from build123d import *

# Parameters (mm, degrees)
BOSS_EXTRUDE3_DEPTH = 4
SKETCH2_W           = 40
SKETCH2_H           = 36.696145016
SKETCH2_W_2         = 20
SKETCH2_H_2         = 40
BOSS_EXTRUDE4_DEPTH = 2
LOFT8_START         = -60
LOFT8_DEPTH         = 40
SKETCH10_W          = 24
SKETCH10_H          = 13
CUT_EXTRUDE1_DEPTH  = 6
SKETCH11_W          = 20
SKETCH11_H          = 40
BOSS_EXTRUDE5_DEPTH = 4


# Read off the part's stored shape, not the designer's step: Loft8
with BuildPart() as part:
    # Sketch1 → Boss-Extrude3 (new body)
    with BuildSketch(Plane(origin=(0, 0, 0), x_dir=(1, 0, 0), z_dir=(0, 1, 0))):
        with BuildLine():
            Line((-55, -30), (55, -30))
            ThreePointArc((55, -30), (62.071067812, -27.071067812), (65, -20))
            Line((65, -20), (65, 20))
            ThreePointArc((65, 20), (62.071067812, 27.071067812), (55, 30))
            Line((55, 30), (-55, 30))
            ThreePointArc((-55, 30), (-62.071067812, 27.071067812), (-65, 20))
            Line((-65, 20), (-65, -20))
            ThreePointArc((-65, -20), (-62.071067812, -27.071067812), (-55, -30))
        make_face()
    extrude(amount=-BOSS_EXTRUDE3_DEPTH)

    # Sketch2 → Boss-Extrude4 (add)
    with BuildSketch(Plane(origin=(0, 2, 0), x_dir=(1, 0, 0), z_dir=(0, 1, 0))):
        with Locations((-40, 1.651927492)):
            Rectangle(SKETCH2_W, SKETCH2_H)
        with Locations((48.333333333, 0)):
            Rectangle(SKETCH2_W_2, SKETCH2_H_2)
    extrude(amount=-BOSS_EXTRUDE4_DEPTH)

    # Loft8 outline → Loft8 (add)
    with BuildSketch(Plane.YZ.offset(LOFT8_START)):
        with BuildLine():
            Line((92.073834687, -4.303854984), (92.073834687, 1.696145016))
            Line((92.073834687, 1.696145016), (12.073834687, 1.696145016))
            ThreePointArc((12.073834687, 1.696145016), (5.064409277, 7.871430337), (2, 16.696145016))
            Line((2, 16.696145016), (2, -20))
            ThreePointArc((2, -20), (4.932872822, -10.801545174), (12.073834687, -4.303854984))
            Line((12.073834687, -4.303854984), (92.073834687, -4.303854984))
        make_face()
    extrude(amount=LOFT8_DEPTH)

    # Sketch10 → Cut-Extrude1 (cut)
    with BuildSketch(Plane.XY.offset(1.696145016)):
        with Locations((-41.946023743, 83.186487073)):
            Rectangle(SKETCH10_W, SKETCH10_H)
    extrude(amount=-CUT_EXTRUDE1_DEPTH, mode=Mode.SUBTRACT)

    # Sketch11 → Boss-Extrude5 (add)
    # profile 1 of 5: a face of its own
    with BuildSketch(Plane(origin=(0, 2, 0), x_dir=(1, 0, 0), z_dir=(0, 1, 0))):
        with Locations((48.333333333, 0)):
            Rectangle(SKETCH11_W, SKETCH11_H)
        Polygon((57.333333333, 2), (57.333333333, 0), (57.333333333, -2), (57.333333333, -17.5), (50.333333333, -17.5), (48.333333333, -17.5), (46.333333333, -17.5), (39.333333333, -17.5), (39.333333333, -2), (39.333333333, 0), (39.333333333, 2), (39.333333333, 17.5), (46.333333333, 17.5), (48.333333333, 17.5), (50.333333333, 17.5), (57.333333333, 17.5), align=None, mode=Mode.SUBTRACT)
    # profile 2 of 5: a face of its own
    with BuildSketch(Plane(origin=(0, 2, 0), x_dir=(1, 0, 0), z_dir=(0, 1, 0))):
        Polygon((50.333333333, 17.5), (57.333333333, 2), (57.333333333, 17.5), align=None)
    # profile 3 of 5: a face of its own
    with BuildSketch(Plane(origin=(0, 2, 0), x_dir=(1, 0, 0), z_dir=(0, 1, 0))):
        Polygon((39.333333333, 2), (46.333333333, 17.5), (39.333333333, 17.5), align=None)
    # profile 4 of 5: a face of its own
    with BuildSketch(Plane(origin=(0, 2, 0), x_dir=(1, 0, 0), z_dir=(0, 1, 0))):
        Polygon((39.333333333, -17.5), (46.333333333, -17.5), (39.333333333, -2), align=None)
    # profile 5 of 5: a face of its own
    with BuildSketch(Plane(origin=(0, 2, 0), x_dir=(1, 0, 0), z_dir=(0, 1, 0))):
        Polygon((57.333333333, -17.5), (57.333333333, -2), (50.333333333, -17.5), align=None)
    extrude(amount=BOSS_EXTRUDE5_DEPTH)


solid = part.part
CAD build for the part. Positions are in the model's coordinates, mm. A direction names the side the tool comes from. Coordinates: 2 decimals unless noted, no trailing zeros. Loops run counter-clockwise (first coordinate to the right, second up) from the corner with the lowest first, then second, coordinate; pieces in that order, holes last. Notation, with made-up numbers: (-3, 32.25) -> (33, 32.25) arc R19 cw to (33, 64.25) -> close; hole circle Ø9 at (49.5, -36.5). An arc over 180 degrees is marked (long way). One line per item, written item: value.
1. Slice it at B-B on x = -23.5. Write the cut outline in (y, z).
Answers:
outline: (-4, -30) -> (0, -30) -> (0, -20) -> (2, -20) arc R18.64 cw to (12.07, -4.3) -> (92.07, -4.3) -> (92.07, 1.7) -> (12.07, 1.7) arc R18.36 cw to (2, 16.7) -> (0, 16.7) -> (0, 30) -> (-4, 30) -> close
2. Pull direction Z, two halves, no side cores. Call faces 5 (the face through (48, 2, 0)), 6 (the face through (-61.99, -1.97, -27.15)), 7 (the face through (-53.946, 83, -1)): pulls with the +Z half, pulls with the -Z half, needs draft (parallel to the pull), parting line crosses it, or undercut.
Answers:
face 5: undercut
face 6: pulls with the -Z half
face 7: needs draft
3. Slice it at D-D on y = 68.5. Write the cut outline in (x, z).
Answers:
outline: (-60, -4.3) -> (-20, -4.3) -> (-20, 1.7) -> (-60, 1.7) -> close
4. Slice it at C-C on z = 6.5. Write the cut outline in (x, y), and give its area (4 significant figures).
Answers:
outline: (-65, -4) -> (65, -4) -> (65, 0) -> (58.33, 0) -> (58.33, 6) -> (55.3, 6) -> (55.3, 2) -> (41.37, 2) -> (41.37, 6) -> (38.33, 6) -> (38.33, 0) -> (-20, 0) -> (-20, 6.08) -> (-60, 6.08) -> (-60, 0) -> (-65, 0) -> close
area: 827.5 mm^2
5. Slice it at A-A on x = -38. Write the cut outline in (y, z).
Answers:
outline: (-4, -30) -> (0, -30) -> (0, -20) -> (2, -20) arc R18.64 cw to (12.07, -4.3) -> (76.69, -4.3) -> (76.69, 1.7) -> (12.07, 1.7) arc R18.36 cw to (2, 16.7) -> (0, 16.7) -> (0, 30) -> (-4, 30) -> close; (89.69, -4.3) -> (92.07, -4.3) -> (92.07, 1.7) -> (89.69, 1.7) -> close
6. Flat gauge pins, fed straight in: P1, Ø3, axis at y = 81, z = -2, coming from the -X side; P2, Ø1, axis at x = -25.5, z = 14.5, coming from the +Y side; P3, Ø1.8, axis at x = 44.5, y = 4, coming from the -Z side. Where does each tip first touch, or does it go through?
Answers:
P1: stops at x = -60
P2: stops at y = 2.41
P3: stops at z = -20
7. Which spindle directions (+Z, -Z, +X, -X, +Y, -Y) get a long thin tool onto all of the face, cutting with end or side? Do faces 1 (the face through (39.333, 4, 0)), 2 (the face through (48, 3, 20)), 3 (the face through (-60, 36, -2)), 4 (the face through (-42, 76.686, -1)). Say none if no direction does.
Answers:
face 1: +Y
face 2: +Z, +X, -X, +Y
face 3: +Z, -Z, -X, +Y
face 4: +Z, -Z
8. Drill centre lines: line 1 (Y direction, x = -48.5, z = 0); line 2 (X direction, y = 83, z = 1); line 3 (Y direction, x = 45.5, z = -15.5). Where is each one in solid material? Low to high. Write a range as [from, to].
Answers:
line 1: y = [-4, 76.69], [89.69, 92.07]
line 2: x = [-60, -53.95], [-29.95, -20]
line 3: y = [-4, 2]
